```python
from build123d import *

# Parameters (mm, degrees)
F2_DEPTH = 5
F3_DEPTH = 5
F4_W     = 13.9
F4_H     = 19.2
F4_R     = 4.75
F5_DEPTH = 10


with BuildPart() as f2:
    # F1 (on offset) → F2 (new body)
    with BuildSketch(Plane.XY.offset(2.5)):
        with BuildLine():
            Line((45, 35), (-45, 35))
            ThreePointArc((-45, 35), (-55.6066017178, 30.6066017178), (-60, 20))
            Line((-60, 20), (-60, -20))
            ThreePointArc((-60, -20), (-55.6066017178, -30.6066017178), (-45, -35))
            Line((-45, -35), (45, -35))
            ThreePointArc((45, -35), (55.6066017178, -30.6066017178), (60, -20))
            Line((60, -20), (60, 20))
            ThreePointArc((60, 20), (55.6066017178, 30.6066017178), (45, 35))
        make_face()
        with BuildLine():
            Line((-45, 30), (45, 30))
            ThreePointArc((45, 30), (52.0710678119, 27.0710678119), (55, 20))
            Line((55, 20), (55, -20))
            ThreePointArc((55, -20), (52.0710678119, -27.0710678119), (45, -30))
            Line((45, -30), (-45, -30))
            ThreePointArc((-45, -30), (-52.0710678119, -27.0710678119), (-55, -20))
            Line((-55, -20), (-55, 20))
            ThreePointArc((-55, 20), (-52.0710678119, 27.0710678119), (-45, 30))
        make_face(mode=Mode.SUBTRACT)
        with BuildLine():
            ThreePointArc((55, 20), (52.0710678119, 27.0710678119), (45, 30))
            Line((45, 30), (-45, 30))
            ThreePointArc((-45, 30), (-52.0710678119, 27.0710678119), (-55, 20))
            Line((-55, 20), (-55, -20))
            ThreePointArc((-55, -20), (-52.0710678119, -27.0710678119), (-45, -30))
            Line((-45, -30), (45, -30))
            ThreePointArc((45, -30), (52.0710678119, -27.0710678119), (55, -20))
            Line((55, -20), (55, 20))
        make_face()
        with BuildLine():
            Line((-45, 29), (45, 29))
            ThreePointArc((45, 29), (51.3639610307, 26.3639610307), (54, 20))
            Line((54, 20), (54, -20))
            ThreePointArc((54, -20), (51.3639610307, -26.3639610307), (45, -29))
            Line((45, -29), (-45, -29))
            ThreePointArc((-45, -29), (-51.3639610307, -26.3639610307), (-54, -20))
            Line((-54, -20), (-54, 20))
            ThreePointArc((-54, 20), (-51.3639610307, 26.3639610307), (-45, 29))
        make_face(mode=Mode.SUBTRACT)
        with BuildLine():
            ThreePointArc((54, 20), (51.3639610307, 26.3639610307), (45, 29))
            Line((45, 29), (-45, 29))
            ThreePointArc((-45, 29), (-51.3639610307, 26.3639610307), (-54, 20))
            Line((-54, 20), (-54, -20))
            ThreePointArc((-54, -20), (-51.3639610307, -26.3639610307), (-45, -29))
            Line((-45, -29), (45, -29))
            ThreePointArc((45, -29), (51.3639610307, -26.3639610307), (54, -20))
            Line((54, -20), (54, 20))
        make_face()
    extrude(amount=F2_DEPTH)

    # F1 (on offset) → F3 (join)
    with BuildSketch(Plane.XY.offset(2.5)):
        with BuildLine():
            ThreePointArc((54, 20), (51.3639610307, 26.3639610307), (45, 29))
            Line((45, 29), (-45, 29))
            ThreePointArc((-45, 29), (-51.3639610307, 26.3639610307), (-54, 20))
            Line((-54, 20), (-54, -20))
            ThreePointArc((-54, -20), (-51.3639610307, -26.3639610307), (-45, -29))
            Line((-45, -29), (45, -29))
            ThreePointArc((45, -29), (51.3639610307, -26.3639610307), (54, -20))
            Line((54, -20), (54, 20))
        make_face()
    extrude(amount=-F3_DEPTH)

    # F4 (on face) → F5 (cut, through all)
    with BuildSketch(Plane.XY.offset(7.5)):
        with Locations((-30, -8.75)):
            Rectangle(F4_W, F4_H)
        with Locations((30, -8.75)):
            Circle(F4_R)
    extrude(amount=-F5_DEPTH, mode=Mode.SUBTRACT)


solid = f2.part
```
CAD build for the part. Positions are in the model's coordinates, mm. A direction names the side the tool comes from. Round coordinates to 2 decimals unless told otherwise and drop trailing zeros. Order: outer loops, then holes, each group sorted by start corner. A loop starts at its lowest first (then second) coordinate and runs counter-clockwise, first axis right, second up. Notation, with made-up numbers: (21.5, 25.25) - (70.5, 25.25) arc R10 cw to (70.5, 42.25) - close; hole circle Ø1 at (-29, 49). An arc over 180 degrees is marked (long way). Answer as CSV lines item,"result". Start each with the question number.
1. Pin check, flat tips, straight feed: pin 1 (5 mm diameter, centred on x = -27.5, z = 0.5, fed in from +Y); pin 2 (4 mm diameter, centred on y = 6.5, z = 0, fed in from -X); pin 3 (1 mm diameter, centred on x = -18, z = 1.5, fed in from +Y); pin 4 (2.5 mm diameter, centred on y = 8, z = 0, fed in from +X). Stop position of each tip, or through.
2. Saw through at B-B, the plane x = 30. Write the cut outline in (y, z).
3. Saw through at C-C, the plane z = -0.5. Write the cut outline in (x, y), and give its area (3 significant figures).
4. Tool access for faces 4 (the face through (-51.294, 26.434, 0.035)), 5 (the face through (4, 31, 2.5)), 6 (the face through (54, 0, 0)), 7 (the face through (1, 29, 0)), 8 (the face through (-1, -29, 0)): list every direction of +Z, -Z, +X, -X, +Y, -Y with a clear straight run to the whole face (end or side of a thin tool).
5. Drill centre lines: L1, parallel to X at y = -9, z = -1; L2, parallel to Y at x = 30, z = 4.75; L3, parallel to Y at x = 30, z = 1.5. Where is each one in solid material? Low to high. Write a range as [from, to].
6. Pull direction X, two halves, no side cores. Call faces 1 (the face through (-51.434, -26.294, 0.035)), 2 (the face through (34.53, -7.32, 2.57)), 3 (the face through (55.72, 30.49, 4.96)): +X half, -X half, draft (parallel to the pull), parting line (faces both ways), or undercut.
7. Saw through at D-D, the plane x = -2.5. Write the cut outline in (y, z).
8. Saw through at A-A, the plane y = -8.75. Write the cut outline in (x, z).
Model answer:
1,pin 1,"stops at y = 35"
1,pin 2,"stops at x = -54"
1,pin 3,"stops at y = 29"
1,pin 4,"stops at x = 54"
2,outline,"(-35, 2.5) - (-29, 2.5) - (-29, -2.5) - (-13.5, -2.5) - (-13.5, 7.5) - (-35, 7.5) - close; (-4, -2.5) - (29, -2.5) - (29, 2.5) - (35, 2.5) - (35, 7.5) - (-4, 7.5) - close"
3,outline,"(-54, -20) arc R9 ccw to (-45, -29) - (45, -29) arc R9 ccw to (54, -20) - (54, 20) arc R9 ccw to (45, 29) - (-45, 29) arc R9 ccw to (-54, 20) - close; hole (-36.95, -18.35) - (-23.05, -18.35) - (-23.05, 0.85) - (-36.95, 0.85) - close; hole circle Ø9.5 at (30, -8.75)"
3,area,"5,860 mm²"
4,face 4,"-Z, -X, +Y"
4,face 5,"-Z"
4,face 6,"-Z, +X, +Y, -Y"
4,face 7,"-Z, +X, -X, +Y"
4,face 8,"-Z, +X, -X, -Y"
5,L1,"x = [-54, -36.95], [-23.05, 25.26], [34.74, 54]"
5,L2,"y = [-35, -13.5], [-4, 35]"
5,L3,"y = [-29, -13.5], [-4, 29]"
6,face 1,"-X half"
6,face 2,"undercut"
6,face 3,"+X half"
7,outline,"(-35, 2.5) - (-29, 2.5) - (-29, -2.5) - (29, -2.5) - (29, 2.5) - (35, 2.5) - (35, 7.5) - (-35, 7.5) - close"
8,outline,"(-60, 2.5) - (-54, 2.5) - (-54, -2.5) - (-36.95, -2.5) - (-36.95, 7.5) - (-60, 7.5) - close; (-23.05, -2.5) - (25.25, -2.5) - (25.25, 7.5) - (-23.05, 7.5) - close; (34.75, -2.5) - (54, -2.5) - (54, 2.5) - (60, 2.5) - (60, 7.5) - (34.75, 7.5) - close"
